from build123d import *

# Parameters (mm, degrees)
F2_SIZE2 = 1.5748
F2_SIZE  = 1.5748
F4_DEPTH = 12.7
F5_R     = 76.2
F6_DEPTH = 44.451
F8_ANGLE = 180


with BuildPart() as f1:
    # F0 (on Front) → F1 (revolve)
    with BuildSketch(Plane.XZ):
        Polygon((98.425, 0), (0, 0), (0, -44.45), (93.726, -44.45), (98.425, -38.8499498684), align=None)
    revolve(axis=Axis((0, 0, -22.225), (0, 0, 1)))

    # F2
    f2_edges = [f1.edges().sort_by_distance(p)[0] for p in [
        (-98.425, 0, 0),
    ]]
    chamfer(f2_edges, length=F2_SIZE, length2=F2_SIZE2)

    # F3 (on face) → F4 (cut)
    with BuildSketch(Plane(origin=(0, 0, -44.45), x_dir=(1, 0, 0), z_dir=(0, 0, -1))):
        with BuildLine():
            ThreePointArc((-18.5894131096, 85.8708059571), (-18.6203916237, 86.3931713593), (-18.7128928876, 86.9082138798))
            ThreePointArc((-18.7128928876, 86.9082138798), (-23.0090131096, 85.8708059571), (-27.2482663209, 84.6211674612))
            ThreePointArc((-27.2482663209, 84.6211674612), (-22.3777205201, 81.4965250075), (-18.5894131096, 85.8708059571))
        make_face()
        with BuildLine():
            ThreePointArc((-27.2482663209, 84.6211674612), (-23.0090131096, 85.8708059571), (-18.7128928876, 86.9082138798))
            ThreePointArc((-18.7128928876, 86.9082138798), (-24.1528897613, 90.139811739), (-27.2482663209, 84.6211674612))
        make_face()
        with BuildLine():
            ThreePointArc((59.6599475589, 65.9082745736), (62.8617928475, 62.8617928475), (65.9082745736, 59.6599475589))
            ThreePointArc((65.9082745736, 59.6599475589), (66.923633243, 61.1198638129), (67.2813928475, 62.8617928475))
            ThreePointArc((67.2813928475, 62.8617928475), (64.5022179025, 66.9656775679), (59.6599475589, 65.9082745736))
        make_face()
        with BuildLine():
            ThreePointArc((59.6599475589, 65.9082745736), (59.7366637174, 59.7366637174), (65.9082745736, 59.6599475589))
            ThreePointArc((65.9082745736, 59.6599475589), (62.8617928475, 62.8617928475), (59.6599475589, 65.9082745736))
        make_face()
        with BuildLine():
            ThreePointArc((-86.9082138798, 18.7128928876), (-85.8708059571, 23.0090131096), (-84.6211674612, 27.2482663209))
            ThreePointArc((-84.6211674612, 27.2482663209), (-90.139811739, 24.1528897613), (-86.9082138798, 18.7128928876))
        make_face()
        with BuildLine():
            ThreePointArc((-81.4512059571, 23.0090131096), (-82.3313309638, 25.6557055609), (-84.6211674612, 27.2482663209))
            ThreePointArc((-84.6211674612, 27.2482663209), (-85.8708059571, 23.0090131096), (-86.9082138798, 18.7128928876))
            ThreePointArc((-86.9082138798, 18.7128928876), (-83.1369500625, 19.5364209787), (-81.4512059571, 23.0090131096))
        make_face()
        with BuildLine():
            ThreePointArc((-65.9082745736, -59.6599475589), (-62.8617928475, -62.8617928475), (-59.6599475589, -65.9082745736))
            ThreePointArc((-59.6599475589, -65.9082745736), (-58.757908127, -64.5022179025), (-58.4421928475, -62.8617928475))
            ThreePointArc((-58.4421928475, -62.8617928475), (-61.1198638129, -58.799952452), (-65.9082745736, -59.6599475589))
        make_face()
        with BuildLine():
            ThreePointArc((-65.9082745736, -59.6599475589), (-65.9869219776, -65.9869219776), (-59.6599475589, -65.9082745736))
            ThreePointArc((-59.6599475589, -65.9082745736), (-62.8617928475, -62.8617928475), (-65.9082745736, -59.6599475589))
        make_face()
        with BuildLine():
            ThreePointArc((18.7128928876, -86.9082138798), (23.0090131096, -85.8708059571), (27.2482663209, -84.6211674612))
            ThreePointArc((27.2482663209, -84.6211674612), (21.8651364579, -81.6018001752), (18.7128928876, -86.9082138798))
        make_face()
        with BuildLine():
            ThreePointArc((27.4286131096, -85.8708059571), (27.3832940593, -85.2395133675), (27.2482663209, -84.6211674612))
            ThreePointArc((27.2482663209, -84.6211674612), (23.0090131096, -85.8708059571), (18.7128928876, -86.9082138798))
            ThreePointArc((18.7128928876, -86.9082138798), (23.5313785118, -90.259427443), (27.4286131096, -85.8708059571))
        make_face()
        with BuildLine():
            ThreePointArc((84.6211674612, -27.2482663209), (85.8708059571, -23.0090131096), (86.9082138798, -18.7128928876))
            ThreePointArc((86.9082138798, -18.7128928876), (81.6018001752, -21.8651364579), (84.6211674612, -27.2482663209))
        make_face()
        with BuildLine():
            ThreePointArc((90.2904059571, -23.0090131096), (89.343398088, -20.275157215), (86.9082138798, -18.7128928876))
            ThreePointArc((86.9082138798, -18.7128928876), (85.8708059571, -23.0090131096), (84.6211674612, -27.2482663209))
            ThreePointArc((84.6211674612, -27.2482663209), (88.5174984084, -26.5484881029), (90.2904059571, -23.0090131096))
        make_face()
    extrude(amount=-F4_DEPTH, mode=Mode.SUBTRACT)

    # F5 (on face) → F6 (cut, through all)
    with BuildSketch(Plane.XY):
        Circle(F5_R)
    extrude(amount=-F6_DEPTH, mode=Mode.SUBTRACT)


with BuildPart() as f1_1:
    # F8: moved
    add(f1.part.rotate(Axis((4.3097957969, 0, 0), (-1, 0, 0)), F8_ANGLE))


with BuildPart() as f1_2:
    # F9: moved
    add(f1_1.part.moved(Location((0, 0, -44.45))))


solid = f1_2.part
Can you work these out from the model? Positions are in its coordinate system, mm. A direction names the side the tool comes from. Round coordinates to 2 decimals unless told otherwise and drop trailing zeros. Loops run counter-clockwise (first coordinate to the right, second up) from the corner with the lowest first, then second, coordinate; pieces in that order, holes last. Notation, with made-up numbers: (4.25, 74) - (25.25, 74) arc R24 cw to (25.25, 110) - close; hole circle Ø11 at (78.5, 48). An arc over 180 degrees is marked (long way). Use CSV: the item, a comma, the result in double quotes. Start each with the question number.
1) If we section it at D-D on z = -39: Write out the boundary of the cut face in (x, y) (3 decimals), plus the area to 3 significant figures.
2) For pin 1 Ø5 at (y, z) = (45.5, -37.5) entering from +X; pin 2 Ø1.5 at (y, z) = (17.5, -29) entering from +X; pin 3 Ø2.5 at (x, y) = (-63, -63) entering from +Z, each with a flat end and sliding along its axis, tell me the tip position at first contact or that it passes through.
3) We'd pull the mould along Z, two halves only. Please class faces 3 (the cylindrical face through (93.88, -29.56, -24.5)), 4 (the flat face through (-63, -63, -12.7)), 5 (the flat face through (-58, 50, -44.45)): released by +Z, released by -Z, zero draft, split by the parting line, or undercut.
4) Please list where these lines run through material, in increasing order: probe 1 along X at (y, z) = (0, -26) (3 decimals); probe 2 along X at (y, z) = (-22, -5). Write a range as [from, to].
5) For faces 1 (the flat face through (0, -77, 0)), 2 (the flat face through (-86, 23, -12.7)), which set-ups out of +Z, -Z, +X, -X, +Y, -Y let a thin tool reach every point of the face, with its end or its side?
6) If we section it at A-A on y = 0: Write out the boundary of the cut face in (x, z) (3 decimals), plus the area to 3 significant figures.
7) If we section it at C-C on z = -9.5: Write out the boundary of the cut face in (x, y) (3 decimals).
Geometry results:
1,outline,"circle Ø196.85 at (0, 0); hole circle Ø152.4 at (0, 0)"
1,area,"12,200 mm2"
2,pin 1,"stops at x = 88.54"
2,pin 2,"stops at x = 96.99"
2,pin 3,"stops at z = -12.7"
3,face 3,"zero draft"
3,face 4,"released by +Z"
3,face 5,"released by -Z"
4,probe 1,"x = [-98.425, -76.2], [76.2, 98.425]"
4,probe 2,"x = [-95.42, -72.96], [72.96, 81.57], [90.17, 95.42]"
5,face 1,"+Z, +X, -X, +Y, -Y"
5,face 2,"+Z"
6,outline,"(-98.425, -42.875) - (-96.85, -44.45) - (-76.2, -44.45) - (-76.2, 0) - (-93.726, 0) - (-98.425, -5.6) - close; (76.2, -44.45) - (96.85, -44.45) - (98.425, -42.875) - (98.425, -5.6) - (93.726, 0) - (76.2, 0) - close"
6,area,"1,950 mm2"
7,outline,"circle Ø196.85 at (0, 0); hole circle Ø8.839 at (-85.871, 23.009); hole circle Ø152.4 at (0, 0); hole circle Ø8.839 at (-62.862, -62.862); hole circle Ø8.839 at (-23.009, 85.871); hole circle Ø8.839 at (23.009, -85.871); hole circle Ø8.839 at (62.862, 62.862); hole circle Ø8.839 at (85.871, -23.009)"
